Geometry check sheet. Reference: drawing and pictorial views, mm from the part's lowest x, y, z. Round coordinates to 2 decimals unless told otherwise and drop trailing zeros. Write each loop counter-clockwise with the first axis right and the second up, starting at its lowest first coordinate (ties: lowest second). Pieces come first, ordered by that corner, then holes. Notation, with made-up numbers: M 81.5,-39.75 L 132.5,-39.75 A20 ccw 132.5,-24.75 Z; hole C 70,33.5 d2. An arc over 180 degrees is marked long. One line per item, written item: value. Start each with the question number.
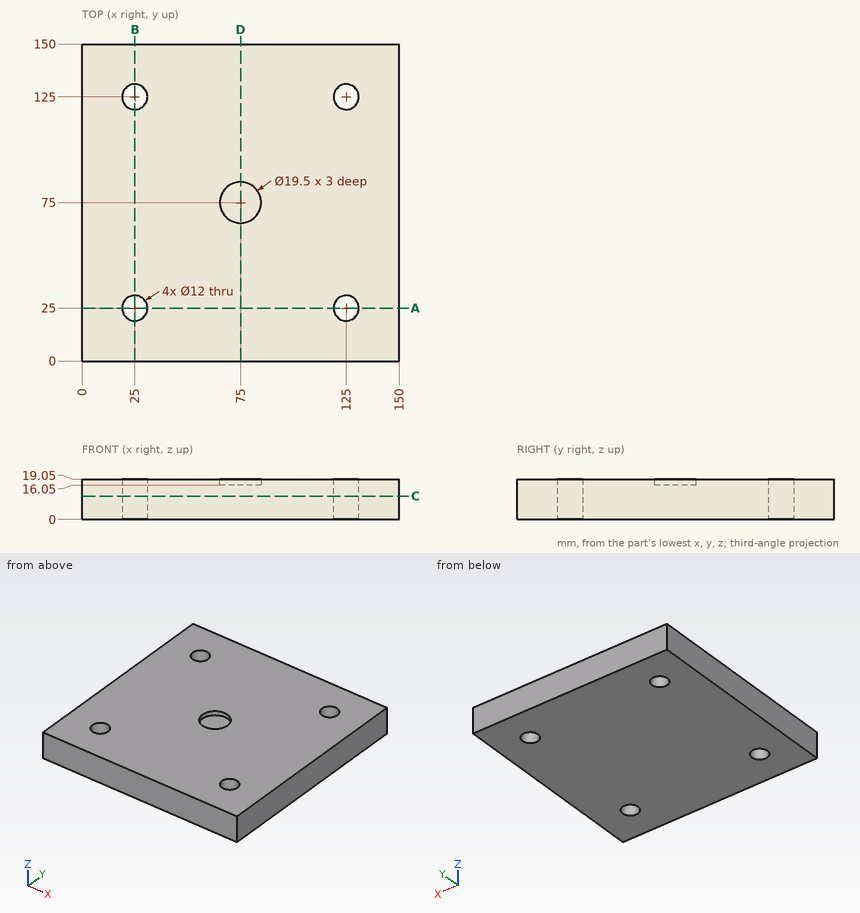
1) Cross-section at A-A (y = 25). Record the boundary of the cut face in (x, z), then the cut area to 3 significant figures.
2) Cross-section at D-D (x = 75). Record the boundary of the cut face in (y, z).
3) Thickness scan on line 1 (Y direction, x = 25, z = 6); line 2 (X direction, y = 22.5, z = 9.5). Record the ranges inside material, lowest first.
4) Cross-section at C-C (z = 11). Record the boundary of the cut face in (x, y).
Results below:
1. outline: M 0,0 L 19,0 L 19,19.05 L 0,19.05 Z; M 31,0 L 119,0 L 119,19.05 L 31,19.05 Z; M 131,0 L 150,0 L 150,19.05 L 131,19.05 Z
1. area: 2,400 mm²
2. outline: M 0,0 L 150,0 L 150,19.05 L 84.75,19.05 L 84.75,16.05 L 65.25,16.05 L 65.25,19.05 L 0,19.05 Z
3. line 1: y = 0 to 19, 31 to 119, 131 to 150
3. line 2: x = 0 to 19.55, 30.45 to 119.55, 130.45 to 150
4. outline: M 0,0 L 150,0 L 150,150 L 0,150 Z; hole C 25,25 d12; hole C 25,125 d12; hole C 125,25 d12; hole C 125,125 d12
